Verification items for the finished model (mm, model axes). Face numbers are marked on the shaded views. A direction names the side the tool comes from. Give positions to 0.01 mm unless a question says otherwise; leave off trailing zeros. Loops run counter-clockwise (first coordinate to the right, second up) from the corner with the lowest first, then second, coordinate; pieces in that order, holes last. Notation, with made-up numbers: M 53,21 L 73,21 A21 cw 73,25 Z; hole C 87.5,12.5 d7. An arc over 180 degrees is marked long. Answer in a Markdown table with one row per item.
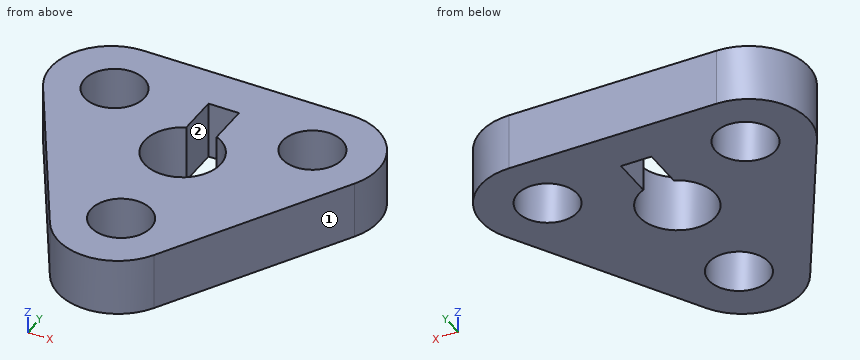
```python
from build123d import *

# Parameters (mm, degrees)
SKETCH2_R           = 6.35
SKETCH2_R_2         = 5
BOSS_EXTRUDE1_DEPTH = 9.525
FILLET1_R           = 10
SKETCH3_W           = 5.08
SKETCH3_H           = 12.7
CUT_EXTRUDE1_DEPTH  = 42.678960958


with BuildPart() as part:
    # Sketch2 → Boss-Extrude1 (new body)
    with BuildSketch(Plane.XY):
        Polygon((-34.641016151, 20), (0, -40), (34.641016151, 20), align=None)
        with Locations(Location((0, 0, 0), (0, 0, 180))):
            Circle(SKETCH2_R, mode=Mode.SUBTRACT)
        with Locations(Location((-16.497783942, 9.525, 0), (0, 0, 180))):
            Circle(SKETCH2_R_2, mode=Mode.SUBTRACT)
        with Locations(Location((16.497783942, 9.525, 0), (0, 0, 180))):
            Circle(SKETCH2_R_2, mode=Mode.SUBTRACT)
        with Locations(Location((0, -19.05, 0), (0, 0, 180))):
            Circle(SKETCH2_R_2, mode=Mode.SUBTRACT)
    extrude(amount=BOSS_EXTRUDE1_DEPTH)

    # Fillet1
    fillet1_edges = [part.edges().sort_by_distance(p)[0] for p in [
        (34.641016151, 20, 4.7625),
        (0, -40, 4.7625),
        (-34.641016151, 20, 4.7625),
    ]]
    fillet(fillet1_edges, radius=FILLET1_R)

    # Sketch3 → Cut-Extrude1 (cut, through all)
    with BuildSketch(Plane.XY):
        with Locations((0, 6.35)):
            Rectangle(SKETCH3_W, SKETCH3_H)
    extrude(amount=CUT_EXTRUDE1_DEPTH, mode=Mode.SUBTRACT)


solid = part.part
```
Item 1: Tool access check on the marked faces 1 and 2. Record the directions out of +Z, -Z, +X, -X, +Y, -Y that give a thin tool (end or side, any length) a straight path to the whole face; none if there is none.
Reported:
| item | result |
|---|---|
| face 1 | +Z, -Z, +X, -Y |
| face 2 | +Z, -Z |
Item 2: Sectioned sample at C-C (x = -19). Record the cut outline in (y, z) (3 decimals).
Reported:
| item | result |
|---|---|
| outline | M -7.091,0 L 5.196,0 L 5.196,9.525 L -7.091,9.525 Z; M 13.854,0 L 19.858,0 L 19.858,9.525 L 13.854,9.525 Z |
Item 3: Go/stop test with flat-tipped pins: pin 1 (1.5 mm diameter, centred on y = -8, z = 5.5, fed in from +X); pin 2 (6 mm diameter, centred on x = 16.5, y = 9.52, fed in from -Z); pin 3 (3 mm diameter, centred on x = 5.5, z = 2, fed in from -Y); pin 4 (1.5 mm diameter, centred on y = -1.5, z = 6.5, fed in from -X). Record where each tip stops, or that it passes through.
Reported:
| item | result |
|---|---|
| pin 1 | stops at x = 18.91 |
| pin 2 | passes through |
| pin 3 | stops at y = -29.17 |
| pin 4 | stops at x = -22.66 |
Item 4: Sectioned sample at D-D (y = -19.05). Record the cut outline in (x, z) (3 decimals), and give its area (3 significant figures).
Reported:
| item | result |
|---|---|
| outline | M -12.095,0 L -5,0 L -5,9.525 L -12.095,9.525 Z; M 5,0 L 12.095,0 L 12.095,9.525 L 5,9.525 Z |
| area | 135 mm^2 |
Item 5: Sectioned sample at A-A (x = 0). Record the cut outline in (y, z) (3 decimals), and give its area (3 significant figures).
Reported:
| item | result |
|---|---|
| outline | M -30,0 L -24.05,0 L -24.05,9.525 L -30,9.525 Z; M -14.05,0 L -6.35,0 L -6.35,9.525 L -14.05,9.525 Z; M 12.7,0 L 20,0 L 20,9.525 L 12.7,9.525 Z |
| area | 200 mm^2 |
Item 6: Sectioned sample at B-B (z = 3.25). State how many separate pieces and enclosed holes the cut face has, and give its area (3 significant figures).
Reported:
| item | result |
|---|---|
| separate pieces | 1 |
| enclosed holes | 4 |
| area | 1,480 mm^2 |
Item 7: Scan lines: L1, parallel to Y at x = 0, z = 4.75; L2, parallel to X at y = 11, z = 5; L3, parallel to X at y = 14, z = 5.5. Record each from-to range of solid material in increasing order. Write a range as [from, to].
Reported:
| item | result |
|---|---|
| L1 | y = [-30, -24.05], [-14.05, -6.35], [12.7, 20] |
| L2 | x = [-27.27, -21.28], [-11.72, -2.54], [2.54, 11.72], [21.28, 27.27] |
| L3 | x = [-26.49, -18.73], [-14.27, 14.27], [18.73, 26.49] |
